Work out the finished part from the listing and answer in its coordinate system (mm). A direction names the side the tool comes from. Round coordinates to 2 decimals unless told otherwise and drop trailing zeros. Write each loop counter-clockwise with the first axis right and the second up, starting at its lowest first coordinate (ties: lowest second). Pieces come first, ordered by that corner, then holes. Notation, with made-up numbers: (31, -37) -> (55, -37) arc R11 ccw to (55, -32) -> close; hole circle Ø8 at (16.25, -16.5). An arc over 180 degrees is marked (long way). One line per item, written item: value.
```python
from build123d import *

# Parameters (mm, degrees)
F0_W     = 2.832651
F0_H     = 6.35
F0_R     = 1.905
F1_DEPTH = 12.7
F2_DEPTH = 38.1
F3_DEPTH = 31.75


with BuildPart() as f1:
    # F0 (on Front) → F1 (new body)
    with BuildSketch(Plane.XZ):
        with Locations((49.418978, -5.683978)):
            Rectangle(F0_W, F0_H)
        Polygon((14.173562, -8.858978), (48.002653, -8.858978), (48.002653, -2.508978), (14.173562, -2.508978), (14.173562, -5.683978), align=None)
        with Locations((41.669869, -5.683978)):
            Circle(F0_R, mode=Mode.SUBTRACT)
        with Locations((23.338998, -5.683978)):
            Circle(F0_R, mode=Mode.SUBTRACT)
        with BuildLine():
            Line((10.998562, -8.858978), (14.173562, -8.858978))
            Line((14.173562, -8.858978), (14.173562, -5.683978))
            ThreePointArc((14.173562, -5.683978), (13.243626, -7.929042), (10.998562, -8.858978))
        make_face()
        with BuildLine():
            Line((14.173562, -5.683978), (14.173562, -2.508978))
            Line((14.173562, -2.508978), (10.998562, -2.508978))
            ThreePointArc((10.998562, -2.508978), (13.243626, -3.438914), (14.173562, -5.683978))
        make_face()
        with BuildLine():
            ThreePointArc((10.998562, -8.858978), (13.243626, -7.929042), (14.173562, -5.683978))
            ThreePointArc((14.173562, -5.683978), (13.243626, -3.438914), (10.998562, -2.508978))
            ThreePointArc((10.998562, -2.508978), (7.823562, -5.683978), (10.998562, -8.858978))
        make_face()
        with Locations((10.998562, -5.683978)):
            Circle(F0_R, mode=Mode.SUBTRACT)
        with Locations((23.338998, -5.683978)):
            Circle(F0_R)
        with Locations((41.669869, -5.683978)):
            Circle(F0_R)
        with Locations((10.998562, -5.683978)):
            Circle(F0_R)
    extrude(amount=F1_DEPTH)

    # F0 (on Front) → F2 (join)
    with BuildSketch(Plane.XZ):
        with Locations((23.338998, -5.683978)):
            Circle(F0_R)
        with Locations((41.669869, -5.683978)):
            Circle(F0_R)
    extrude(amount=F2_DEPTH)

    # F0 (on Front) → F3 (join)
    with BuildSketch(Plane.XZ):
        with Locations((10.998562, -5.683978)):
            Circle(F0_R)
    extrude(amount=-F3_DEPTH)


solid = f1.part
```
(1) Find section C-C on y = -4. Give the vertices of the cut face in (x, z) (3 decimals), plus the area to 3 significant figures.
Reported:
outline: (10.999, -8.859) -> (50.835, -8.859) -> (50.835, -2.509) -> (10.999, -2.509) arc R3.175 ccw to start
area: 269 mm2
(2) Flat-ended cylindrical pins translate along their axes: pin 1 Ø3 at (y, z) = (-23.5, -4) entering from +X; pin 2 Ø3 at (y, z) = (12, -3.5) entering from -X; pin 3 Ø4 at (x, y) = (41.5, 2.5) entering from +Z; pin 4 Ø1.9 at (x, z) = (34, -6.5) entering from +Y. Find the tip coordinate at first contact, or state that the pin passes through.
Reported:
pin 1: stops at x = 43.57
pin 2: stops at x = 9.22
pin 3: passes through
pin 4: stops at y = 0
(3) Find section B-B on y = -23.5. Give the vertices of the cut face in (x, z) (3 decimals), plus the area to 3 significant figures.
Reported:
outline: circle Ø3.81 at (23.339, -5.684); circle Ø3.81 at (41.67, -5.684)
area: 22.8 mm2
(4) Consider probe 1 along Y at (x, z) = (42, -4); probe 2 along Y at (x, z) = (27.5, -4); probe 3 along X at (y, z) = (-26.5, -5.5). Determine where each line is inside the solid, lowest interval first.
Reported:
probe 1: y = -38.1 to 0
probe 2: y = -12.7 to 0
probe 3: x = 21.44 to 25.24, 39.77 to 43.57
(5) For a pull along X with two mould halves and no side action, classify faces 4 (the face through (11, 31.75, -6)), 5 (the face through (7.824, -6.261, -5.614)), 6 (the face through (41.257, -25.222, -7.544)) as pulls with the +X half, pulls with the -X half, needs draft (parallel to the pull), parting line crosses it, or undercut.
Reported:
face 4: needs draft
face 5: pulls with the -X half
face 6: undercut
(6) A tool of negligible diameter and unlimited length cuts with its end or side. For faces 1 (the face through (10.586, 15.653, -7.544)), 2 (the face through (21.827, -25.222, -6.843)), 3 (the face through (50.835, -6, -6)), from which of +Z, -Z, +X, -X, +Y, -Y can it reach the whole face along a straight path? Write none if from no direction.
Reported:
face 1: +Y
face 2: -Y
face 3: +Z, -Z, +X, +Y, -Y
(7) Find section D-D on z = -6.5. Give the vertices of the cut face in (x, y).
Reported:
outline: (7.93, -12.7) -> (21.62, -12.7) -> (21.62, -38.1) -> (25.06, -38.1) -> (25.06, -12.7) -> (39.95, -12.7) -> (39.95, -38.1) -> (43.39, -38.1) -> (43.39, -12.7) -> (50.84, -12.7) -> (50.84, 0) -> (12.72, 0) -> (12.72, 31.75) -> (9.28, 31.75) -> (9.28, 0) -> (7.93, 0) -> close
(8) Find section A-A on x = 24. Give the vertices of the cut face in (y, z).
Reported:
outline: (-38.1, -7.47) -> (-12.7, -7.47) -> (-12.7, -8.86) -> (0, -8.86) -> (0, -2.51) -> (-12.7, -2.51) -> (-12.7, -3.9) -> (-38.1, -3.9) -> close
